Input: dimensioned drawing with shaded views. Units: mm. Origin: part minimum x, y, z. Give positions to 0.01 mm unless a question says otherwise; leave off trailing zeros. Write each loop counter-clockwise with the first axis right and the second up, starting at its lowest first coordinate (ties: lowest second). Pieces come first, ordered by that corner, then holes.
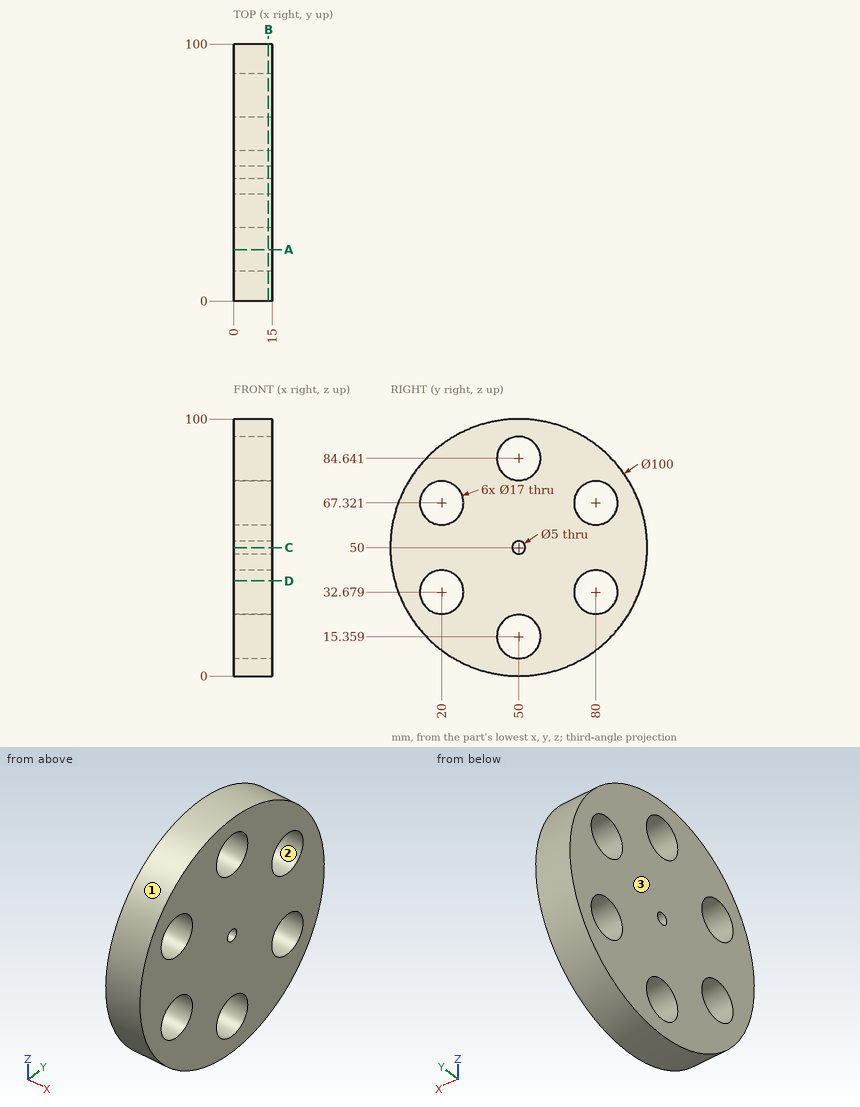
Item 1: Pin query (flat end, axial travel): pin 1 (15.5 mm diameter, centred on y = 20, z = 32.68, fed in from -X); pin 2 (1 mm diameter, centred on x = 3, y = 70, fed in from +Z); pin 3 (2 mm diameter, centred on x = 3.5, y = 71, fed in from +Z) (1 decimal); pin 4 (2 mm diameter, centred on x = 8, z = 27, fed in from -Y). Return the tip coordinate at first contact, or that it passes through.
Item 2: Section D-D (z = 37). Return loops of the section in (x, y), and give its area (3 significant figures).
Item 3: Mould query, pull axis Y, two halves, no side actions, for the marked faces 1, 2 and 3. Classes: +Y half, -Y half, draft (parallel to the pull), parting line (faces both ways), or undercut.
Item 4: Section A-A (y = 20). Return loops of the section in (x, z), and give its area (3 significant figures).
Item 5: Ray query, line 1 (Z direction, x = 5.75, y = 81); line 2 (Y direction, x = 11.25, z = 50); line 3 (Z direction, x = 11.5, y = 84). Return the intervals inside material, ascending.
Item 6: Section B-B (x = 13.5). Return loops of the section in (y, z).
Item 7: Section C-C (z = 50). Return loops of the section in (x, y), and give its area (4 significant figures).
Solved:
1. pin 1: passes through
1. pin 2: stops at z = 96.04
1. pin 3: stops at z = 95.8
1. pin 4: stops at y = 5.1
2. outline: (0, 1.72) - (15, 1.72) - (15, 12.68) - (0, 12.68) - close; (0, 27.32) - (15, 27.32) - (15, 72.68) - (0, 72.68) - close; (0, 87.32) - (15, 87.32) - (15, 98.28) - (0, 98.28) - close
2. area: 1,010 mm2
3. face 1: parting line
3. face 2: undercut
3. face 3: draft
4. outline: (0, 10) - (15, 10) - (15, 24.18) - (0, 24.18) - close; (0, 41.18) - (15, 41.18) - (15, 58.82) - (0, 58.82) - close; (0, 75.82) - (15, 75.82) - (15, 90) - (0, 90) - close
4. area: 690 mm2
5. line 1: z = 10.77 to 24.24, 41.12 to 58.88, 75.76 to 89.23
5. line 2: y = 0 to 47.5, 52.5 to 100
5. line 3: z = 13.34 to 25.18, 40.18 to 59.82, 74.82 to 86.66
6. outline: circle Ø100 at (50, 50); hole circle Ø17 at (20, 32.68); hole circle Ø17 at (20, 67.32); hole circle Ø17 at (50, 15.36); hole circle Ø17 at (50, 84.64); hole circle Ø5 at (50, 50); hole circle Ø17 at (80, 32.68); hole circle Ø17 at (80, 67.32)
7. outline: (0, 0) - (15, 0) - (15, 47.5) - (0, 47.5) - close; (0, 52.5) - (15, 52.5) - (15, 100) - (0, 100) - close
7. area: 1,425 mm2
